Autodesk Inventor part; units mm, degrees
ref_plane "YZ Plane" through (0, 0, 0) normal (1, 0, 0) x (0, 1, 0)
ref_plane "XZ Plane" through (0, 0, 0) normal (0, 1, 0) x (-1, 0, 0)
ref_plane "XY Plane" through (0, 0, 0) normal (0, 0, 1) x (1, 0, 0)
sketch "Sketch1" plane through (0, 0, 0) normal (0, 1, 0) x (-1, 0, 0)
  line L0 (50.8, 25.4) -> (-50.8, 25.4)
  line L1 (-50.8, 25.4) -> (-50.8, -25.4)
  line L2 (-50.8, -25.4) -> (50.8, -25.4)
  line L3 (50.8, -25.4) -> (50.8, 25.4)
  line L4 (50.8, 25.4) -> (-50.8, -25.4) construction
  line L5 (-50.8, 25.4) -> (50.8, -25.4) construction
  point P0 (0, 0)
  dimension "d0" = 101.6
  dimension "d1" = 50.8
extrude "Extrusion1" add sketch "Sketch1" along normal blind 3.175
sketch "Sketch3" plane through (0, 3.175, 0) normal (0, 1, 0) x (1, 0, 0)
  line L0 (50.8, 25.4) -> (-50.8, 25.4)
  line L1 (0, 25.4) -> (0, 22.098) construction
  line L2 (-50.8, 25.4) -> (-50.8, -25.4) construction
  line L3 (-50.8, 25.4) -> (-50.8, -25.4) construction
  line L4 (-50.8, 25.4) -> (-47.498, 25.4) construction
  line L5 (-47.498, 25.4) -> (-47.498, -25.4) construction
  line L6 (-50.8, -25.4) -> (50.8, -25.4) construction
  line L7 (-47.498, 22.098) -> (50.8, 22.098) construction
  line L8 (50.8, -25.4) -> (50.8, 25.4)
  line L9 (-47.498, 22.098) -> (50.8, 22.098)
  line L10 (50.8, 22.098) -> (50.8, 19.558)
  line L11 (50.8, 19.558) -> (-47.498, 19.558)
  line L12 (-47.498, 19.558) -> (-47.498, 22.098)
  point P0 (0, 0)
  dimension "d8" = 3.302
  dimension "d9" = 3.302
  dimension "d10" = 2.54
extrude "Extrusion3" add sketch "Sketch3" against normal blind 25.4
sketch "Sketch4" plane through (0, 3.175, 0) normal (0, 1, 0) x (1, 0, 0)
  line L0 (50.8, 19.558) -> (-47.498, 19.558)
  line L1 (-50.8, -25.4) -> (50.8, -25.4)
  line L2 (50.8, 19.558) -> (48.26, 19.558)
  line L3 (48.26, 19.558) -> (48.26, -25.4)
  line L4 (48.26, -25.4) -> (50.8, -25.4)
  line L5 (50.8, -25.4) -> (50.8, 19.558)
  point P0 (0, 0)
  dimension "d13" = 2.54
extrude "Extrusion4" add sketch "Sketch4" against normal blind 9.525
sketch "Sketch5" plane through (-50.8, 3.175, 25.4) normal (0, 0, 1) x (1, 0, 0)
  line L0 (101.6, -3.175) -> (0, -3.175)
  line L1 (101.6, -3.175) -> (76.2, -3.175)
  line L2 (76.2, -3.175) -> (76.2, -1.651)
  line L3 (76.2, -1.651) -> (101.6, -1.651)
  line L4 (101.6, -1.651) -> (101.6, -3.175)
  point P0 (50.8, -3.175)
  dimension "d16" = 25.4
  dimension "d17" = 1.524
extrude "Extrusion5" add sketch "Sketch5" along normal blind 3.175
properties part number "Wire Housing Wall vglue"
Could you check a few things on this model? Use its own coordinates, in mm. A direction names the side the tool comes from. Give positions to 0.01 mm unless a question says otherwise; leave off trailing zeros. Order: outer loops, then holes, each group sorted by start corner. A loop starts at its lowest first (then second) coordinate and runs counter-clockwise, first axis right, second up. Notation, with made-up numbers: (85, -11) -> (128, -11) arc R17 ccw to (128, 20) -> close; hole circle Ø10 at (-36.75, -16.5). An arc over 180 degrees is marked (long way). Answer in a Markdown table with one row per item. Add a question column.
Item 1: Imagine slicing it at D-D (x = -32.5). List the corners of the cut face in (y, z) for me (3 decimals).
Item 2: For faces 1 (the flat face through (1, -11, -22.098)), 2 (the flat face through (38, 1.524, 27)), 3 (the flat face through (-47.498, -11, -21)), 4 (the flat face through (48.26, -3, 3)), 5 (the flat face through (50, -3, 25.4)), which set-ups out of +Z, -Z, +X, -X, +Y, -Y let a thin tool reach every point of the face, with its end or its side?
Item 3: Imagine slicing it at A-A (x = 40). List the corners of the cut face in (y, z) for me (3 decimals), and give its area (3 significant figures).
Item 4: Please list where these lines run through material, in increasing order: probe 1 along Y at (x, z) = (15.5, 11) (3 decimals); probe 2 along Z at (x, y) = (-20.5, -4.5); probe 3 along X at (y, z) = (-5, 19.5).
Item 5: I'm going to push flat-ended pins straight in: P1, Ø2, axis at x = 49, z = 5, coming from the -Y side; P2, Ø0.8, axis at y = -8.5, z = -21, coming from the -X side; P3, Ø16, axis at x = 23.5, z = 4.5, coming from the -Y side. Where does each tip first touch, or does it pass through?
Item 6: Imagine slicing it at B-B (z = -21). List the corners of the cut face in (x, y) for me (3 decimals).
Item 7: Imagine slicing it at C-C (y = -3.5). List the corners of the cut face in (x, z) for me, and give its area (3 significant figures).
Result:
| question | item | result |
|---|---|---|
| 1 | outline | (-22.225, -22.098) -> (0, -22.098) -> (0, -25.4) -> (3.175, -25.4) -> (3.175, 25.4) -> (0, 25.4) -> (0, -19.558) -> (-22.225, -19.558) -> close |
| 2 | face 1 | -Z, +X, -X, -Y |
| 2 | face 2 | +Z, +X, -X, +Y |
| 2 | face 3 | +Z, -Z, -X, -Y |
| 2 | face 4 | +Z, -X, -Y |
| 2 | face 5 | +Z, +X, -X, -Y |
| 3 | outline | (-22.225, -22.098) -> (0, -22.098) -> (0, -25.4) -> (3.175, -25.4) -> (3.175, 25.4) -> (1.524, 25.4) -> (1.524, 28.575) -> (0, 28.575) -> (0, -19.558) -> (-22.225, -19.558) -> close |
| 3 | area | 223 mm2 |
| 4 | probe 1 | 0 to 3.175 |
| 4 | probe 2 | -22.1 to -19.56 |
| 4 | probe 3 | 48.26 to 50.8 |
| 5 | P1 | y = -6.35 |
| 5 | P2 | x = -47.5 |
| 5 | P3 | y = 0 |
| 6 | outline | (-50.8, 0) -> (-47.498, 0) -> (-47.498, -22.225) -> (50.8, -22.225) -> (50.8, 3.175) -> (-50.8, 3.175) -> close |
| 7 | outline | (-47.5, -22.1) -> (50.8, -22.1) -> (50.8, 25.4) -> (48.26, 25.4) -> (48.26, -19.56) -> (-47.5, -19.56) -> close |
| 7 | area | 364 mm2 |
